Source: CAD feature listing. Evaluate the final solid. Frame: model axes, mm. Face numbers are marked on the shaded views. A direction names the side the tool comes from. Coordinates: 2 decimals unless noted, no trailing zeros. Loops run counter-clockwise (first coordinate to the right, second up) from the corner with the lowest first, then second, coordinate; pieces in that order, holes last.
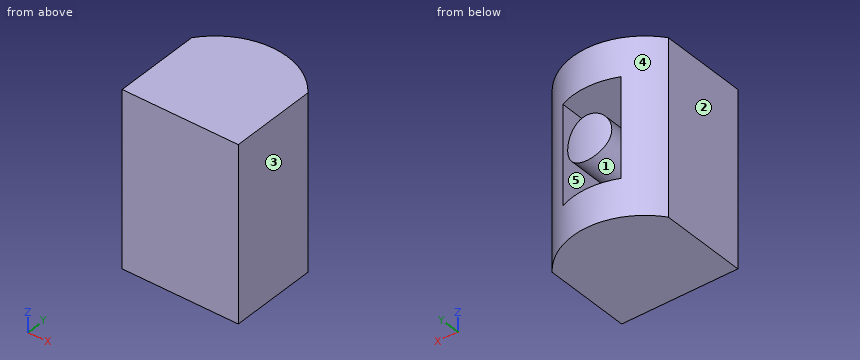
Autodesk Inventor part; units mm, degrees
ref_plane "YZ Plane" through (0, 0, 0) normal (1, 0, 0) x (0, 1, 0)
ref_plane "XZ Plane" through (0, 0, 0) normal (0, 1, 0) x (-1, 0, 0)
ref_plane "XY Plane" through (0, 0, 0) normal (0, 0, 1) x (1, 0, 0)
sketch "Sketch1" plane through (0, 0, 0) normal (0, 1, 0) x (-1, 0, 0)
  line L0 (169.4818, -66.9774) -> (67.8818, -66.9774)
  line L1 (67.8818, -66.9774) -> (67.8818, -219.3774)
  line L2 (67.8818, -219.3774) -> (169.4818, -219.3774)
  line L3 (169.4818, -219.3774) -> (169.4818, -66.9774)
  point P0 (0, 0)
  dimension "d0" = 152.4
  dimension "d1" = 101.6
extrude "Extrusion1" add sketch "Sketch1" along normal blind 101.6
sketch "Sketch2" plane through (0, 101.6, 0) normal (0, 1, 0) x (1, 0, 0)
  line L0 (-144.0818, 99.9974) -> (-93.2818, 99.9974)
  line L1 (-93.2818, 99.9974) -> (-93.2818, 186.3574)
  line L2 (-93.2818, 186.3574) -> (-144.0818, 186.3574)
  line L3 (-144.0818, 186.3574) -> (-144.0818, 99.9974)
  circle A0 centre (-118.6818, 143.1774) radius 19.2808
  line L4 (-67.8818, 219.3774) -> (-169.4818, 219.3774)
  line L5 (-169.4818, 66.9774) -> (-67.8818, 66.9774)
  line L6 (-169.4818, 219.3774) -> (-169.4818, 66.9774)
  line L7 (-67.8818, 66.9774) -> (-67.8818, 219.3774)
  point P0 (0, 0)
  dimension "d4" = 33.02
  dimension "d5" = 33.02
  dimension "d6" = 76.2
  dimension "d7" = 50.8
  dimension "d8" = 25.4
  dimension "d9" = 25.4
extrude "Extrusion2" cut sketch "Sketch2" against normal blind 63.5 contours L3 L2 L1 L0
sketch "Sketch3" plane through (-169.4818, 0, -66.9774) normal (0, 0, 1) x (1, 0, 0)
  line L0 (101.6, 0) -> (0, 0)
  arc A0 (101.6, 0) -> (0, 0) centre (50.8, 38.1) ccw
  line L1 (76.2, 101.6) -> (25.4, 101.6)
  point P0 (169.4818, 0)
extrude "Extrusion3" cut sketch "Sketch3" against normal up to surface (152.4 mm away) keep common part
properties part number "complex extrusion 1 5.7.20"
Q1. Material intervals for line 1 along Z through (x, y) = (-119.5, 78.5); line 2 along Z through (x, y) = (-139, 55); line 3 along Z through (x, y) = (-105, 88), sorted ascending.
Q2. Section query D-D on y = 40.5. Return the cut outline in (x, z).
Q3. Section query C-C on x = -131. Return the cut outline in (y, z).
Q4. Reachability of the marked faces 1 and 2 from +Z, -Z, +X, -X, +Y, -Y: full face, straight path, thin tool, end or side. Return the list, or none.
Q5. Section query B-B on z = -122. Return the cut outline in (x, y).
Q6. Draft query along X for the marked faces 3, 4 and 5. Return one class per face: released by +X, released by -X, zero draft, split by the parting line, or undercut.
Q7. Section query A-A on y = 88. Return the cut outline in (x, z), then the cut area to 3 significant figures.
Resolved:
1. line 1: z = -219.38 to -186.36, -162.44 to -123.91, -100 to -66.98
1. line 2: z = -219.38 to -186.36, -100 to -66.98
1. line 3: z = -219.38 to -186.36, -156.76 to -129.59, -100 to -66.98
2. outline: (-169.48, -219.38) - (-67.88, -219.38) - (-67.88, -66.98) - (-169.48, -66.98) - close; circle Ø38.56 at (-118.68, -143.18); hole (-144.08, -186.36) - (-93.28, -186.36) - (-93.28, -100) - (-144.08, -100) - close
3. outline: (0, -219.38) - (100.39, -219.38) - (100.39, -186.36) - (38.1, -186.36) - (38.1, -158.01) - (100.39, -158.01) - (100.39, -128.34) - (38.1, -128.34) - (38.1, -100) - (100.39, -100) - (100.39, -66.98) - (0, -66.98) - close
4. face 1: +Y
4. face 2: +Z, -Z, -X, +Y, -Y
5. outline: (-169.48, 0) - (-67.88, 0) - (-67.88, 76.2) arc R63.5 ccw to (-93.28, 96.3) - (-93.28, 38.1) - (-144.08, 38.1) - (-144.08, 96.3) arc R63.5 ccw to (-169.48, 76.2) - close
6. face 3: released by +X
6. face 4: split by the parting line
6. face 5: undercut
7. outline: (-157.95, -219.38) - (-79.41, -219.38) - (-79.41, -66.98) - (-157.95, -66.98) - close; circle Ø38.56 at (-118.68, -143.18); hole (-144.08, -186.36) - (-93.28, -186.36) - (-93.28, -100) - (-144.08, -100) - close
7. area: 8,750 mm2
